Here's how the part is built. I have some questions about the finished solid (model axes, mm). A direction names the side the tool comes from. Coordinates: 2 decimals unless noted, no trailing zeros. Write each loop counter-clockwise with the first axis right and the second up, starting at its lowest first coordinate (ties: lowest second). Pieces come first, ordered by that corner, then holes.
```python
from build123d import *

# Parameters (mm, degrees)
BOSS_EXTRU_1_DEPTH = 25
ESQUISSE2_R        = 25
ESQUISSE2_R_2      = 12.5
BOSS_EXTRU_2_DEPTH = 25


with BuildPart() as part:
    # Esquisse1 → Boss.-Extru.1 (new body)
    with BuildSketch(Plane(origin=(0, 0, 0), x_dir=(0, 1, 0), z_dir=(0, 0, 1))):
        Polygon((19.282032303, 46.602540378), (-30.717967697, 40), (-50, -6.602540378), (-19.282032303, -46.602540378), (30.717967697, -40), (50, 6.602540378), align=None)
    extrude(amount=BOSS_EXTRU_1_DEPTH)

    # Esquisse2 → Boss.-Extru.2 (add)
    with BuildSketch(Plane(origin=(0, 0, 0), x_dir=(0, 1, 0), z_dir=(0, 0, 1))):
        with Locations(Location((0, 0, 0), (0, 0, 270))):
            Circle(ESQUISSE2_R)
        with Locations(Location((0, 0, 0), (0, 0, 270))):
            Circle(ESQUISSE2_R_2, mode=Mode.SUBTRACT)
    extrude(amount=-BOSS_EXTRU_2_DEPTH)


solid = part.part
```
1) Will these pins go through, and if not, where does the flat tip stop? pin 1 (2 mm diameter, centred on x = -4.5, z = 2.5, fed in from +Y); pin 2 (6 mm diameter, centred on x = -1.5, z = 12.5, fed in from +Y); pin 3 (1 mm diameter, centred on x = -22, y = -38, fed in from -Z).
Values follow:
pin 1: stops at y = 49.54
pin 2: stops at y = 49.13
pin 3: stops at z = 0
2) I need wall thicknesses on probe 1 along Y at (x, z) = (0, -5.5); probe 2 along Z at (x, y) = (-35, -5.5); probe 3 along X at (y, z) = (-10, -12). Which ranges of each line are inside material? Lowest first, please.
Values follow:
probe 1: y = -25 to -12.5, 12.5 to 25
probe 2: z = 0 to 25
probe 3: x = -22.91 to -7.5, 7.5 to 22.91
3) Imagine slicing it at C-C on y = -17. Please give me the cut outline in (x, z).
Values follow:
outline: (-41.81, 0) - (-18.33, 0) - (-18.33, -25) - (18.33, -25) - (18.33, 0) - (46.3, 0) - (46.3, 25) - (-41.81, 25) - close
4) Imagine slicing it at A-A on z = 15. Please give me the cut outline in (x, y).
Values follow:
outline: (-46.6, 19.28) - (-40, -30.72) - (6.6, -50) - (46.6, -19.28) - (40, 30.72) - (-6.6, 50) - close
5) Imagine slicing it at B-B on x = 8. Please give me the cut outline in (y, z), then the cut area to 3 significant figures.
Values follow:
outline: (-48.93, 0) - (-23.69, 0) - (-23.69, -25) - (-9.6, -25) - (-9.6, 0) - (9.6, 0) - (9.6, -25) - (23.69, -25) - (23.69, 0) - (43.96, 0) - (43.96, 25) - (-48.93, 25) - close
area: 3,030 mm2
6) We'd pull the mould along X, two halves only. Please class faces 3 (the face through (23.846, 7.509, -12.325)), 4 (the face through (11.923, 3.755, -12.325)), 5 (the face through (-11.5, 5.9, -25)), 6 (the face through (0, 0, 0)): pulls with the +X half, pulls with the -X half, needs draft (parallel to the pull), parting line crosses it, or undercut.
Values follow:
face 3: parting line crosses it
face 4: undercut
face 5: needs draft
face 6: undercut
7) On a 3-axis mill with a long thin cutter (end or side, diameter ignored), from which of +Z, -Z, +X, -X, +Y, -Y can I reach the whole of each face in a straight line? I mean faces 1 (the face through (-11, -23, 0)), 2 (the face through (-43.347, -5.368, 12.325)). Say none if no direction works.
Values follow:
face 1: -Z
face 2: +Z, -Z, -X, -Y
8) Imagine slicing it at D-D on x = 19. Please give me the cut outline in (y, z).
Values follow:
outline: (-40.48, 0) - (-16.25, 0) - (-16.25, -25) - (16.25, -25) - (16.25, 0) - (39.41, 0) - (39.41, 25) - (-40.48, 25) - close
